from build123d import *

# Parameters (mm, degrees)
SKETCH_1_W              = 80
SKETCH_1_H              = 80
EXTRUDE_1_DEPTH         = 140
SKETCH_2_OUTSIDE_W      = 118
SKETCH_2_OUTSIDE_H      = 118
CUT_EXTRUDE_1_DEPTH     = 129
HOLE_WIZARD_6_5_6_5_1_D = 6.5


with BuildPart() as part:
    # 草图1 → 凸台-拉伸1 (new body)
    with BuildSketch(Plane.XY):
        Rectangle(SKETCH_1_W, SKETCH_1_H)
    extrude(amount=EXTRUDE_1_DEPTH)

    # 草图2 outside → 切除-拉伸1 (cut)
    with BuildSketch(Plane.XY.offset(140)):
        Rectangle(SKETCH_2_OUTSIDE_W, SKETCH_2_OUTSIDE_H)
        with BuildLine():
            Line((30, 25), (35, 25))
            ThreePointArc((35, 25), (38.535533906, 23.535533906), (40, 20))
            Line((40, 20), (40, -20))
            ThreePointArc((40, -20), (38.535533906, -23.535533906), (35, -25))
            Line((35, -25), (30, -25))
            ThreePointArc((30, -25), (26.464466094, -26.464466094), (25, -30))
            Line((25, -30), (25, -35))
            ThreePointArc((25, -35), (23.535533906, -38.535533906), (20, -40))
            Line((20, -40), (-20, -40))
            ThreePointArc((-20, -40), (-23.535533906, -38.535533906), (-25, -35))
            Line((-25, -35), (-25, -30))
            ThreePointArc((-25, -30), (-26.464466094, -26.464466094), (-30, -25))
            Line((-30, -25), (-35, -25))
            ThreePointArc((-35, -25), (-38.535533906, -23.535533906), (-40, -20))
            Line((-40, -20), (-40, 20))
            ThreePointArc((-40, 20), (-38.535533906, 23.535533906), (-35, 25))
            Line((-35, 25), (-30, 25))
            ThreePointArc((-30, 25), (-26.464466094, 26.464466094), (-25, 30))
            Line((-25, 30), (-25, 35))
            ThreePointArc((-25, 35), (-23.535533906, 38.535533906), (-20, 40))
            Line((-20, 40), (20, 40))
            ThreePointArc((20, 40), (23.535533906, 38.535533906), (25, 35))
            Line((25, 35), (25, 30))
            ThreePointArc((25, 30), (26.464466094, 26.464466094), (30, 25))
        make_face(mode=Mode.SUBTRACT)
    extrude(amount=-CUT_EXTRUDE_1_DEPTH, mode=Mode.SUBTRACT)

    # Ø6.5 (6.5) 直径孔1 (through all)
    with Locations(Plane(origin=(-31.75, 31.75, 11), x_dir=(1, 0, 0), z_dir=(0, 0, 1))):
        with Locations((0, 0), (63.5, 0), (63.5, -63.5), (0, -63.5)):
            Hole(HOLE_WIZARD_6_5_6_5_1_D / 2)


solid = part.part
Geometry: final body of the model. Coordinates: model frame, mm. A direction names the side the tool comes from. Round coordinates to 2 decimals unless told otherwise and drop trailing zeros. Order: outer loops, then holes, each group sorted by start corner. A loop starts at its lowest first (then second) coordinate and runs counter-clockwise, first axis right, second up.
Q1. Section A-A, the plane x = -31.75. Output: boundary loops of the cut face in (y, z).
Result sheet:
outline: (-40, 0) - (-35, 0) - (-35, 11) - (-40, 11) - close; (-28.5, 0) - (28.5, 0) - (28.5, 11) - (25, 11) - (25, 140) - (-25, 140) - (-25, 11) - (-28.5, 11) - close; (35, 0) - (40, 0) - (40, 11) - (35, 11) - close
Q2. Access query for faces 4 (the face through (33, -25, 76)), 5 (the face through (-35, 35, 11)), 6 (the face through (23, 39, 76)), 7 (the face through (-38, -24, 76)). Directions: +Z, -Z, +X, -X, +Y, -Y. A direction counts if a zero-diameter tool reaches every point of the face in a straight line with its end or side. Return the directions, or none.
Result sheet:
face 4: +Z, +X, -Y
face 5: +Z, -X, +Y
face 6: +Z, +X, +Y
face 7: +Z, -X, -Y
Q3. Material intervals for probe 1 along Y at (x, z) = (31.75, 6.75); probe 2 along X at (y, z) = (31, 4), sorted ascending.
Result sheet:
probe 1: y = -40 to -35, -28.5 to 28.5, 35 to 40
probe 2: x = -40 to -34.91, -28.59 to 28.59, 34.91 to 40
Q4. Mould query, pull axis X, two halves, no side actions, for faces 1 (the face through (-25, -33, 76)), 2 (the face through (-33.25, -34.633, 5.423)), 3 (the face through (34, 35, 11)). Classes: released by +X, released by -X, zero draft, split by the parting line, or undercut.
Result sheet:
face 1: released by -X
face 2: undercut
face 3: zero draft
Q5. Section C-C, the plane z = 35.5. Output: boundary loops of the cut face in (x, y).
Result sheet:
outline: (-40, -20) arc R5 ccw to (-35, -25) - (-30, -25) arc R5 cw to (-25, -30) - (-25, -35) arc R5 ccw to (-20, -40) - (20, -40) arc R5 ccw to (25, -35) - (25, -30) arc R5 cw to (30, -25) - (35, -25) arc R5 ccw to (40, -20) - (40, 20) arc R5 ccw to (35, 25) - (30, 25) arc R5 cw to (25, 30) - (25, 35) arc R5 ccw to (20, 40) - (-20, 40) arc R5 ccw to (-25, 35) - (-25, 30) arc R5 cw to (-30, 25) - (-35, 25) arc R5 ccw to (-40, 20) - close
Q6. Pin query (flat end, axial travel): pin 1 (7.5 mm diameter, centred on x = -31.75, y = -31.75, fed in from -Z); pin 2 (4 mm diameter, centred on y = -33.5, z = 53.5, fed in from -X); pin 3 (8.5 mm diameter, centred on x = -31.75, y = 31.75, fed in from +Z); pin 4 (5.5 mm diameter, centred on x = 32.5, z = 95.5, fed in from -Y). Return the tip coordinate at first contact, or that it passes through.
Result sheet:
pin 1: stops at z = 0
pin 2: stops at x = -25
pin 3: stops at z = 11
pin 4: stops at y = -25.01
